Autodesk Inventor part; units mm, degrees
ref_plane "YZ Plane" through (0, 0, 0) normal (1, 0, 0) x (0, 1, 0)
ref_plane "XZ Plane" through (0, 0, 0) normal (0, 1, 0) x (-1, 0, 0)
ref_plane "XY Plane" through (0, 0, 0) normal (0, 0, 1) x (1, 0, 0)
sketch "Sketch1" plane through (0, 0, 0) normal (0, 1, 0) x (-1, 0, 0)
  circle A0 centre (0, 0) radius 10
  dimension "d0" = 20
extrude "Extrusion1" add sketch "Sketch1" along normal blind 40
sketch "Sketch2" plane through (0, 40, 0) normal (0, 1, 0) x (1, 0, 0)
  circle A0 centre (0, 0) radius 2.25
  dimension "d3" = 4.5
extrude "Extrusion2" add sketch "Sketch2" along normal blind 10
sketch "Sketch3" plane through (0, 50, 0) normal (0, 1, 0) x (1, 0, 0)
  circle A0 centre (0, 0) radius 1
  dimension "d6" = 2
extrude "Extrusion3" cut sketch "Sketch3" against normal through all
sketch "Sketch4" plane through (0, 0, 0) normal (0, -1, 0) x (1, 0, 0)
  circle A0 centre (0, 0) radius 7.9
  dimension "d9" = 15.8
extrude "Extrusion4" cut sketch "Sketch4" against normal blind 10
sketch "Sketch5" plane through (0, 10, 0) normal (0, -1, 0) x (1, 0, 0)
  circle A0 centre (0, 0) radius 6.5
  dimension "d12" = 13
extrude "Extrusion5" cut sketch "Sketch5" against normal blind 28
chamfer "Chamfer2" distance 5 angle 45 1 edges at (-6.5, 38, 0)
chamfer "Chamfer3" distance 1.4 angle 45 1 edges at (-6.5, 10, 0)
sketch "Sketch6" plane through (0, 0, 0) normal (0, -1, 0) x (1, 0, 0)
  line L0 (3.75, -9.2702) -> (-3.75, -9.2702)
  line L1 (-3.75, -9.2702) -> (-3.75, -18.7702)
  line L2 (-3.75, -18.7702) -> (3.75, -18.7702)
  line L3 (3.75, -18.7702) -> (3.75, -9.2702)
  circle A0 centre (0, 0) radius 10
  point P0 (-3.75, -9.2702)
  dimension "d24" = 9.5
  dimension "d25" = 7.5
  dimension "d26" = 3.75
extrude "Extrusion6" add sketch "Sketch6" against normal blind 8 contours L3 L2 L1 A0
sketch "Sketch7" plane through (0, 0, 0) normal (0, -1, 0) x (1, 0, 0)
  line L0 (3.75, -11.2702) -> (2.25, -11.2702)
  line L1 (2.25, -11.2702) -> (2.25, -16.7702)
  line L2 (2.25, -16.7702) -> (3.75, -16.7702)
  line L3 (3.75, -16.7702) -> (3.75, -11.2702)
  line L4 (-3.75, -18.7702) -> (3.75, -18.7702)
  line L5 (3.75, -18.7702) -> (3.75, -9.2702)
  point P0 (0, 0)
  dimension "d29" = 1.5
  dimension "d30" = 5.5
  dimension "d31" = 2
extrude "Extrusion7" cut sketch "Sketch7" against normal through all
sketch "Sketch8" plane through (0, 0, 0) normal (0, -1, 0) x (1, 0, 0)
  line L0 (-0.5, -18.7702) -> (0.5, -18.7702)
  line L1 (0.5, -18.7702) -> (0.5, -7.8842)
  line L2 (0.5, -7.8842) -> (-0.5, -7.8842)
  line L3 (-0.5, -7.8842) -> (-0.5, -18.7702)
  line L4 (-3.75, -18.7702) -> (3.75, -18.7702)
  circle A0 centre (0, 0) radius 7.9
  dimension "d34" = 1
  dimension "d35" = 0.5
extrude "Extrusion8" cut sketch "Sketch8" against normal blind 10 contours L3 A0 L1 L0
sketch "Sketch9" plane through (-3.75, 0, -18.7702) normal (-1, 0, 0) x (0, 0, 1)
  circle A0 centre (4.75, 4) radius 1.65
  line L0 (0, 0) -> (0, 8)
  line L1 (0, 8) -> (9.5, 8)
  point P0 (18.7702, 0)
  dimension "d38" = 3.3
  dimension "d39" = 4.75
  dimension "d40" = 4
extrude "Extrusion9" cut sketch "Sketch9" against normal through all
chamfer "Chamfer4" distance 5 angle 45 1 edges at (10, 40, 0)
sketch "Sketch10" plane through (3.75, 0, -18.7702) normal (1, 0, 0) x (0, 0, -1)
  circle A0 centre (-18.7702, 20) radius 1
  line L0 (0, 0) -> (-2, 0)
  point P0 (-18.7702, 0)
  dimension "d46" = 2
  dimension "d47" = 20
  dimension "d48" = 0
extrude "Extrusion10" cut sketch "Sketch10" along normal through all
properties part number "OMEGAETTE_HOUSING"
Design review of the part built by this model. Coordinates are the model's own, in mm. A direction names the side the tool comes from. Round coordinates to 2 decimals unless told otherwise and drop trailing zeros. Write each loop counter-clockwise with the first axis right and the second up, starting at its lowest first coordinate (ties: lowest second). Pieces come first, ordered by that corner, then holes. Notation, with made-up numbers: M -28.5,-2.5 L 4.5,-2.5 A20 ccw 4.5,5.5 Z; hole C 71,-4.5 d9. An arc over 180 degrees is marked long. One line per item, written item: value. Start each with the question number.
1. Clearance check with flat-ended pins moving along their axes: P1, Ø1, axis at x = 3, y = 15, coming from the -Z side; P2, Ø12, axis at x = 6.5, y = 40.5, coming from the +Z side; P3, Ø1.2, axis at x = 0, z = 0, coming from the -Y side; P4, Ø1, axis at x = -1, y = 28.5, coming from the -Z side. State where each tip first meets the part, or that it passes through.
2. Take a section at D-D on y = 46. State the section outline as (x, z) points.
3. To check wall thickness, follow probe 1 along Z at (x, y) = (0, 18); probe 2 along Z at (x, y) = (0, 40.5). State the ranges of each line that lie inside material, in increasing order. Write a range as from..to.
4. Take a section at B-B on y = 37.5. State the section outline as (x, z) points.
5. Take a section at C-C on y = 4. State the section outline as (x, z) points.
6. Draft analysis for pull direction X (two halves, no side actions). For faces 5 (the face through (-2, 8, -14)), 6 (the face through (-0.29, 44.93, 2.23)), 7 (the face through (-5.158, 22.049, -3.955)), state which applies: pulls with the +X half, pulls with the -X half, needs draft (parallel to the pull), parting line crosses it, or undercut.
7. For faces 1 (the face through (-2.2, 40, -1)), 2 (the face through (3.75, 4, -18)), 3 (the face through (3, 4, -16.77)), 4 (the face through (0.5, 4, -12)), list the 3-axis set-ups (+Z, -Z, +X, -X, +Y, -Y) from which the entire face can be reached by the end or side of a thin tool; tool diameter is ignored.
Computed:
1. P1: stops at z = -9.68
1. P2: stops at z = 9.12
1. P3: passes through
1. P4: stops at z = -9.99
2. outline: C 0,0 d4.5; hole C 0,0 d2
3. probe 1: z = -10..-6.5, 6.5..10
3. probe 2: z = -2.25..-1, 1..2.25
4. outline: C 0,0 d15; hole C 0,0 d4
5. outline: M -3.75,-18.77 L -0.5,-18.77 L -0.5,-15.67 L -3.75,-15.67 Z; M -3.75,-12.37 L -0.5,-12.37 L -0.5,-7.88 A7.9 cw long 0.5,-7.88 L 0.5,-12.37 L 2.25,-12.37 L 2.25,-11.27 L 3.75,-11.27 L 3.75,-9.27 A10 ccw long -3.75,-9.27 Z; M 0.5,-18.77 L 3.75,-18.77 L 3.75,-16.77 L 2.25,-16.77 L 2.25,-15.67 L 0.5,-15.67 Z
6. face 5: needs draft
6. face 6: parting line crosses it
6. face 7: undercut
7. face 1: +Y
7. face 2: -Z, +X, +Y, -Y
7. face 3: +X, +Y, -Y
7. face 4: -Z, -Y
